Design review of the part built by this model. Coordinates are the model's own, in mm. Face numbers are marked on the shaded views. A direction names the side the tool comes from. Give positions to 0.01 mm unless a question says otherwise; leave off trailing zeros. Order: outer loops, then holes, each group sorted by start corner. A loop starts at its lowest first (then second) coordinate and runs counter-clockwise, first axis right, second up. Notation, with made-up numbers: M -6,-16.75 L 21,-16.75 A32 cw 21,15.25 Z; hole C 69.5,-27.75 d9. An arc over 180 degrees is marked long. Answer as a JSON object with one key per item and string values.
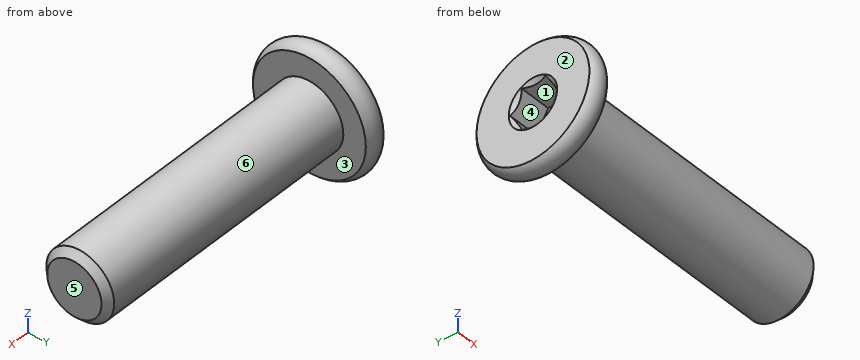
from build123d import *

# Parameters (mm, degrees)
SKETCH2_R           = 2.5
BOSS_EXTRUDE1_DEPTH = 20
CHAMFER1_SIZE       = 0.5
CUT_EXTRUDE1_DEPTH  = 2.3
SKETCH8_R           = 1.782050808
CUT_EXTRUDE2_DEPTH  = 1
CUT_EXTRUDE2_TAPER  = 45


with BuildPart() as part:
    # Sketch2 → Boss-Extrude1 (new body)
    with BuildSketch(Plane(origin=(0, 0, 0), x_dir=(0, 0, -1), z_dir=(1, 0, 0))):
        Circle(SKETCH2_R)
    extrude(amount=-BOSS_EXTRUDE1_DEPTH)

    # Chamfer1
    chamfer1_edges = [part.edges().sort_by_distance(p)[0] for p in [
        (0, 0, 2.5),
    ]]
    chamfer(chamfer1_edges, length=CHAMFER1_SIZE)

    # Sketch6 → Revolve1 (revolve)
    with BuildSketch(Plane.XY):
        with BuildLine():
            Line((-21.5, 0), (-21.5, 4.161437828))
            ThreePointArc((-21.5, 4.161437828), (-20.75, 4.5), (-20, 4.161437828))
            Line((-20, 4.161437828), (-20, 0))
            Line((-20, 0), (-21.5, 0))
        make_face()
    revolve(axis=Axis((-20, 0, 0), (1, 0, 0)))

    # Sketch7 → Cut-Extrude1 (cut)
    with BuildSketch(Plane.ZY.offset(21.5)):
        Polygon((0, 1.732050808), (-1.5, 0.866025404), (-1.5, -0.866025404), (0, -1.732050808), (1.5, -0.866025404), (1.5, 0.866025404), align=None)
    extrude(amount=-CUT_EXTRUDE1_DEPTH, mode=Mode.SUBTRACT)

    # Sketch8 → Cut-Extrude2 (cut)
    with BuildSketch(Plane.ZY.offset(21.5)):
        Circle(SKETCH8_R)
    extrude(amount=-CUT_EXTRUDE2_DEPTH, taper=CUT_EXTRUDE2_TAPER, mode=Mode.SUBTRACT)


solid = part.part
(1) Tool access review of the marked faces 1, 2 and 3: name each direction out of +Z, -Z, +X, -X, +Y, -Y from which nothing blocks a thin tool from reaching the whole face with its end or side.
Checked values:
{"face 1": "-X", "face 2": "+Z, -Z, -X, +Y, -Y", "face 3": "+X"}
(2) Draft analysis for pull direction Y (two halves, no side actions). For the marked faces 4, 5 and 6, state which applies: +Y half, -Y half, draft (parallel to the pull), parting line (faces both ways), or undercut.
Checked values:
{"face 4": "undercut", "face 5": "draft", "face 6": "parting line"}
(3) To check wall thickness, follow L1, parallel to X at y = 1.5, z = 3.5; L2, parallel to Y at x = -2, z = -1.75; L3, parallel to Z at x = -13.5, y = -2. State the ranges of each line that lie inside material, in increasing order. Write a range as from..to.
Checked values:
{"L1": "x = -21.5..-20", "L2": "y = -1.79..1.79", "L3": "z = -1.5..1.5"}
(4) Insertion check: pin 1 (2 mm diameter, centred on x = -17.5, z = -1.5, fed in from -Y); pin 2 (0.9 mm diameter, centred on y = 0, z = 0.5, fed in from -X); pin 3 (1 mm diameter, centred on y = -2.5, z = 3, fed in from +X). Each pin has a flat end and moves straight along its axis. Give the tip position at first contact, or say it passes through.
Checked values:
{"pin 1": "stops at y = -2.45", "pin 2": "stops at x = -19.2", "pin 3": "stops at x = -20"}
(5) We need section A-A (x = -4.75). Write out the cut boundary in (y, z), plus the area to 3 significant figures.
Checked values:
{"outline": "C 0,0 d5", "area": "19.6 mm^2"}
